Could you check a few things on this model? Use its own coordinates, in mm. Face numbers are marked on the shaded views. A direction names the side the tool comes from. Round coordinates to 2 decimals unless told otherwise and drop trailing zeros. Order: outer loops, then holes, each group sorted by start corner. A loop starts at its lowest first (then second) coordinate and runs counter-clockwise, first axis right, second up. Notation, with made-up numbers: M 29.25,48 L 44.25,48 A24 cw 44.25,82 Z; hole C 34,50 d5. An arc over 180 degrees is marked long. Write each question's results on one line, items separated by ' | '. Start each with the question number.
1. For the marked faces 1 and 2, which set-ups out of +Z, -Z, +X, -X, +Y, -Y let a thin tool reach every point of the face, with its end or its side?
2. Suppose I cut it at C-C on x = 48. Write out the boundary of the cut face in (y, z), and give its area (3 significant figures).
3. Please list where these lines run through material, in increasing order: L1, parallel to Y at x = -15.5, z = 3.25; L2, parallel to X at y = 70.25, z = 5; L3, parallel to X at y = -5.5, z = -15.
4. Suppose I cut it at A-A on x = 0. Write out the boundary of the cut face in (y, z), and give its area (3 significant figures).
5. Suppose I cut it at D-D on y = 38. Write out the boundary of the cut face in (x, z), and give its area (3 significant figures).
6. I'm going to push flat-ended pins straight in: pin 1 (5 mm diameter, centred on x = 14.5, z = -24.5, fed in from -Y); pin 2 (5 mm diameter, centred on x = -55.5, y = -22, fed in from -Z); pin 3 (4 mm diameter, centred on x = 67.5, z = 5, fed in from +Y). Where does each tip first touch, or does it pass through?
7. Suppose I cut it at B-B on z = -15. Write out the boundary of the cut face in (x, y).
from build123d import *

# Parameters (mm, degrees)
ESQUISSE1_W             = 165
ESQUISSE1_H             = 150
BOSS_EXTRU_1_DEPTH      = 10
ESQUISSE2_R             = 4.25
ENL_V_MAT_EXTRU_1_DEPTH = 10
ESQUISSE5_W             = 95
ESQUISSE5_H             = 10
BOSS_EXTRU_2_DEPTH      = 5
ESQUISSE4_R             = 1.5
ESQUISSE4_R_2           = 7.5
ENL_V_MAT_EXTRU_2_DEPTH = 15
ESQUISSE6_R             = 1.25
ENL_V_MAT_EXTRU_3_DEPTH = 10
ESQUISSE7_W             = 30
ESQUISSE7_H             = 20
BOSS_EXTRU_3_DEPTH      = 30
ESQUISSE8_R             = 5.5
ESQUISSE8_R_2           = 2
ENL_V_MAT_EXTRU_4_DEPTH = 30
ESQUISSE8_4_R           = 11.5
ESQUISSE8_4_R_2         = 5.5
ESQUISSE8_4_R_3         = 2
ENL_V_MAT_EXTRU_5_DEPTH = 5
ESQUISSE9_R             = 1.25
ENL_V_MAT_EXTRU_6_DEPTH = 15


with BuildPart() as part:
    # Esquisse1 → Boss.-Extru.1 (new body)
    with BuildSketch(Plane.XY):
        Rectangle(ESQUISSE1_W, ESQUISSE1_H)
    extrude(amount=BOSS_EXTRU_1_DEPTH)

    # Esquisse2 → Enl_v. mat.-Extru.1 (cut)
    with BuildSketch(Plane.XY.offset(10)):
        with Locations((-67.5, 60)):
            Circle(ESQUISSE2_R)
        with Locations(Location((67.5, 60, 0), (0, 0, 180))):
            Circle(ESQUISSE2_R)
    extrude(amount=-ENL_V_MAT_EXTRU_1_DEPTH, mode=Mode.SUBTRACT)

    # Esquisse5 → Boss.-Extru.2 (add)
    with BuildSketch(Plane(origin=(0, 75, 0), x_dir=(1, 0, 0), z_dir=(0, 1, 0))):
        with Locations((-15, -5)):
            Rectangle(ESQUISSE5_W, ESQUISSE5_H)
    extrude(amount=BOSS_EXTRU_2_DEPTH)

    # Esquisse4 → Enl_v. mat.-Extru.2 (cut)
    with BuildSketch(Plane.XY.offset(10)):
        with Locations((-15.5, 75.5)):
            Circle(ESQUISSE4_R)
        with Locations((15.5, 75.5)):
            Circle(ESQUISSE4_R)
        with Locations((15.5, 44.5)):
            Circle(ESQUISSE4_R)
        with Locations((-15.5, 44.5)):
            Circle(ESQUISSE4_R)
        with Locations((0, 60)):
            Circle(ESQUISSE4_R_2)
        with Locations((-53, 75.5)):
            Circle(ESQUISSE4_R)
        with Locations((-22, 75.5)):
            Circle(ESQUISSE4_R)
        with Locations((-22, 44.5)):
            Circle(ESQUISSE4_R)
        with Locations((-53, 44.5)):
            Circle(ESQUISSE4_R)
        with Locations((-37.5, 60)):
            Circle(ESQUISSE4_R_2)
    extrude(amount=-ENL_V_MAT_EXTRU_2_DEPTH, mode=Mode.SUBTRACT)

    # Esquisse6 → Enl_v. mat.-Extru.3 (cut)
    with BuildSketch(Plane.XY.offset(10)):
        with Locations((38.715061684, 5)):
            Circle(ESQUISSE6_R)
        with Locations((38.715061684, -5)):
            Circle(ESQUISSE6_R)
        with Locations((53.715061684, -5)):
            Circle(ESQUISSE6_R)
        with Locations((53.715061684, 5)):
            Circle(ESQUISSE6_R)
    extrude(amount=-ENL_V_MAT_EXTRU_3_DEPTH, mode=Mode.SUBTRACT)

    # Esquisse7 → Boss.-Extru.3 (add)
    with BuildSketch(Plane(origin=(0, 0, 0), x_dir=(-1, 0, 0), z_dir=(0, 0, -1))):
        Rectangle(ESQUISSE7_W, ESQUISSE7_H)
    extrude(amount=BOSS_EXTRU_3_DEPTH)

    # Esquisse8 → Enl_v. mat.-Extru.4 (cut)
    with BuildSketch(Plane(origin=(0, 10, 0), x_dir=(1, 0, 0), z_dir=(0, 1, 0))):
        with Locations(Location((0, 15, 0), (0, 0, 270))):
            Circle(ESQUISSE8_R)
        with Locations(Location((-8, 15, 0), (0, 0, 270))):
            Circle(ESQUISSE8_R_2)
        with Locations(Location((0, 23, 0), (0, 0, 270))):
            Circle(ESQUISSE8_R_2)
        with Locations(Location((8, 15, 0), (0, 0, 270))):
            Circle(ESQUISSE8_R_2)
        with Locations(Location((0, 7, 0), (0, 0, 270))):
            Circle(ESQUISSE8_R_2)
    extrude(amount=-ENL_V_MAT_EXTRU_4_DEPTH, mode=Mode.SUBTRACT)

    # Esquisse8_4 → Enl_v. mat.-Extru.5 (cut)
    with BuildSketch(Plane(origin=(0, 10, 0), x_dir=(1, 0, 0), z_dir=(0, 1, 0))):
        with Locations(Location((0, 15, 0), (0, 0, 270))):
            Circle(ESQUISSE8_4_R)
        with Locations(Location((0, 15, 0), (0, 0, 270))):
            Circle(ESQUISSE8_4_R_2, mode=Mode.SUBTRACT)
        with Locations(Location((0, 23, 0), (0, 0, 270))):
            Circle(ESQUISSE8_4_R_3, mode=Mode.SUBTRACT)
        with Locations(Location((8, 15, 0), (0, 0, 270))):
            Circle(ESQUISSE8_4_R_3, mode=Mode.SUBTRACT)
        with Locations(Location((0, 7, 0), (0, 0, 270))):
            Circle(ESQUISSE8_4_R_3, mode=Mode.SUBTRACT)
        with Locations(Location((-8, 15, 0), (0, 0, 270))):
            Circle(ESQUISSE8_4_R_3, mode=Mode.SUBTRACT)
    extrude(amount=-ENL_V_MAT_EXTRU_5_DEPTH, mode=Mode.SUBTRACT)

    # Esquisse9 → Enl_v. mat.-Extru.6 (cut)
    with BuildSketch(Plane(origin=(0, 75, 0), x_dir=(1, 0, 0), z_dir=(0, 1, 0))):
        with Locations(Location((67.5, -5, 0), (0, 0, 270))):
            Circle(ESQUISSE9_R)
        with Locations(Location((-67.5, -5, 0), (0, 0, 270))):
            Circle(ESQUISSE9_R)
    extrude(amount=-ENL_V_MAT_EXTRU_6_DEPTH, mode=Mode.SUBTRACT)


solid = part.part
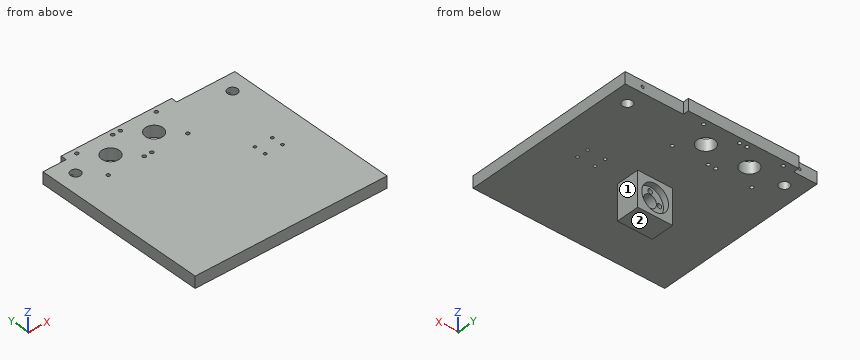
Filled sheet:
1) face 1: -Z, +X, +Y, -Y | face 2: -Z, +X, -X, +Y, -Y
2) outline: M -75,0 L 75,0 L 75,10 L -75,10 Z | area: 1,500 mm^2
3) L1: y = -75 to 43, 46 to 74, 77 to 80 | L2: x = -82.5 to -68.75, -66.25 to 66.25, 68.75 to 82.5 | L3: x = -15 to -10, -6 to -5.5, 5.5 to 6, 10 to 15
4) outline: M -75,0 L -10,0 L -10,-5 L 5,-5 L 5,-3.5 L 10,-3.5 L 10,0 L 52.5,0 L 52.5,10 L -75,10 Z; M -10,-30 L 10,-30 L 10,-26.5 L 5,-26.5 L 5,-25 L -10,-25 Z; M -10,-21 L 5,-21 L 5,-20.5 L -10,-20.5 Z; M -10,-9.5 L 5,-9.5 L 5,-9 L -10,-9 Z; M 67.5,0 L 80,0 L 80,10 L 67.5,10 Z | area: 1,600 mm^2
5) outline: M -82.5,0 L 82.5,0 L 82.5,10 L -82.5,10 Z | area: 1,650 mm^2
6) pin 1: stops at y = -10 | pin 2: stops at z = 0 | pin 3: stops at y = 75
7) outline: M -15,-10 L -10,-10 L -10,5 L -11.5,5 L -11.5,10 L -15,10 Z; M -6,-10 L -5.5,-10 L -5.5,5 L -6,5 Z; M 5.5,-10 L 6,-10 L 6,5 L 5.5,5 Z; M 10,-10 L 15,-10 L 15,10 L 11.5,10 L 11.5,5 L 10,5 Z
